Work out the finished part from the listing and answer in its coordinate system (mm). A direction names the side the tool comes from. Coordinates: 2 decimals unless noted, no trailing zeros. Order: outer loops, then holes, each group sorted by start corner. A loop starts at its lowest first (then second) coordinate and runs counter-clockwise, first axis right, second up. Notation, with made-up numbers: M 61.5,17.5 L 88.5,17.5 A10 ccw 88.5,36.5 Z; hole C 33.25,-7.75 d11. An arc over 180 degrees is marked long. Use a Markdown table: item, result.
from build123d import *

# Parameters (mm, degrees)
SKETCH1_R           = 3.8
SKETCH1_R_2         = 7.5
SKETCH1_R_3         = 6
SKETCH1_W           = 28
SKETCH1_H           = 21
BOSS_EXTRUDE1_DEPTH = 3


with BuildPart() as part:
    # Sketch1 → Boss-Extrude1 (new body)
    with BuildSketch(Plane.XY):
        with BuildLine():
            Line((-44.907534458, -41.831082964), (-44.907534458, -37.831082964))
            Line((-44.907534458, -37.831082964), (-74.907534458, -37.831082964))
            Line((-74.907534458, -37.831082964), (-77.907534458, -37.831082964))
            Line((-77.907534458, -37.831082964), (-77.907534458, 35.317270492))
            ThreePointArc((-77.907534458, 35.317270492), (-78.146852772, 36.26595379), (-78.807534458, 36.987599801))
            ThreePointArc((-78.807534458, 36.987599801), (-78.73201274, 48.728946501), (-68.036732481, 43.883752382))
            ThreePointArc((-68.036732481, 43.883752382), (-67.363200969, 42.667177293), (-66.059360488, 42.183752382))
            Line((-66.059360488, 42.183752382), (77.553779546, 42.183752382))
            Line((77.553779546, 42.183752382), (77.553779546, -37.831082964))
            Line((77.553779546, -37.831082964), (45.092465542, -37.831082964))
            Line((45.092465542, -37.831082964), (45.092465542, -41.831082964))
            Line((45.092465542, -41.831082964), (15.092465542, -41.831082964))
            Line((15.092465542, -41.831082964), (15.092465542, -37.831082964))
            Line((15.092465542, -37.831082964), (-14.907534458, -37.831082964))
            Line((-14.907534458, -37.831082964), (-14.907534458, -41.831082964))
            Line((-14.907534458, -41.831082964), (-44.907534458, -41.831082964))
        make_face()
        with Locations((-74.957534458, 42.833752382)):
            Circle(SKETCH1_R, mode=Mode.SUBTRACT)
        with Locations((-55.663947073, 16.489262872)):
            Circle(SKETCH1_R_2, mode=Mode.SUBTRACT)
        with Locations((-30.663947073, 16.489262872)):
            Circle(SKETCH1_R_2, mode=Mode.SUBTRACT)
        with Locations((-5.663947073, 16.489262872)):
            Circle(SKETCH1_R_2, mode=Mode.SUBTRACT)
        with Locations((54.950876551, -17.44070313)):
            Circle(SKETCH1_R_3, mode=Mode.SUBTRACT)
        with Locations((53.477773965, 15.276803872)):
            Rectangle(SKETCH1_W, SKETCH1_H, mode=Mode.SUBTRACT)
    extrude(amount=BOSS_EXTRUDE1_DEPTH)


solid = part.part
(1) Straight lines are drawn through the part: L1, parallel to Y at x = 40, z = 2.05; L2, parallel to X at y = 21, z = 1.7; L3, parallel to X at y = 20.5, z = 0.35. For each, find the intervals that lie inside material, in ascending order.
Conclusion:
| item | result |
|---|---|
| L1 | -41.83 to 4.78, 25.78 to 42.18 |
| L2 | -77.91 to -61.66, -49.67 to -36.66, -24.67 to -11.66, 0.33 to 39.48, 67.48 to 77.55 |
| L3 | -77.91 to -62, -49.33 to -37, -24.33 to -12, 0.67 to 39.48, 67.48 to 77.55 |
(2) Determine the mould class of faces 4 (the flat face through (53, 4.777, 1)), 5 (the cylindrical face through (-48.51, 18.74, 1.48)), 6 (the flat face through (-77.908, -2, 1)), 7 (the flat face through (62, -37.831, 1)) for opening direction Y: pulls with the +Y half, pulls with the -Y half, needs draft (parallel to the pull), parting line crosses it, or undercut.
Conclusion:
| item | result |
|---|---|
| face 4 | undercut |
| face 5 | undercut |
| face 6 | needs draft |
| face 7 | pulls with the -Y half |
(3) A cutting plane is placed at B-B (x = -30). Determine the outline of the cut face in (y, z).
Conclusion:
| item | result |
|---|---|
| outline | M -41.83,0 L 9.02,0 L 9.02,3 L -41.83,3 Z; M 23.96,0 L 42.18,0 L 42.18,3 L 23.96,3 Z |
(4) A cutting plane is placed at A-A (y = 10.5). Determine the outline of the cut face in (x, z), then the cut area to 3 significant figures.
Conclusion:
| item | result |
|---|---|
| outline | M -77.91,0 L -60.18,0 L -60.18,3 L -77.91,3 Z; M -51.15,0 L -35.18,0 L -35.18,3 L -51.15,3 Z; M -26.15,0 L -10.18,0 L -10.18,3 L -26.15,3 Z; M -1.15,0 L 39.48,0 L 39.48,3 L -1.15,3 Z; M 67.48,0 L 77.55,0 L 77.55,3 L 67.48,3 Z |
| area | 301 mm2 |
(5) A cutting plane is placed at D-D (y = -19). Determine the outline of the cut face in (x, z).
Conclusion:
| item | result |
|---|---|
| outline | M -77.91,0 L 49.16,0 L 49.16,3 L -77.91,3 Z; M 60.74,0 L 77.55,0 L 77.55,3 L 60.74,3 Z |
(6) Given P1, Ø1.5, axis at y = 2, z = 1, coming from the -X side; P2, Ø12, axis at x = 47, y = 16.5, coming from the -Z side; P3, Ø1.5, axis at x = -5, z = 1.5, coming from the -Y side; P4, Ø1.5, axis at y = -39.5, z = 1, coming from the +X side, each flat-ended and moving along its own axis, determine where each tip first touches the part or whether it passes through.
Conclusion:
| item | result |
|---|---|
| P1 | x = -77.91 |
| P2 | through |
| P3 | y = -37.83 |
| P4 | x = 45.09 |
(7) A cutting plane is placed at C-C (z = 0.9). Determine the outline of the cut face in (x, y), then the cut area to 3 significant figures.
Conclusion:
| item | result |
|---|---|
| outline | M -78.81,36.99 A2 cw -77.91,35.32 L -77.91,-37.83 L -44.91,-37.83 L -44.91,-41.83 L -14.91,-41.83 L -14.91,-37.83 L 15.09,-37.83 L 15.09,-41.83 L 45.09,-41.83 L 45.09,-37.83 L 77.55,-37.83 L 77.55,42.18 L -66.06,42.18 A2 cw -68.04,43.88 A7 ccw long Z; hole C -74.96,42.83 d7.6; hole C -55.66,16.49 d15; hole C -30.66,16.49 d15; hole C -5.66,16.49 d15; hole M 39.48,4.78 L 67.48,4.78 L 67.48,25.78 L 39.48,25.78 Z; hole C 54.95,-17.44 d12 |
| area | 11,500 mm2 |
(8) Which of the six approach directions +Z, -Z, +X, -X, +Y, -Y give full straight-line access (tool end or side, diameter ignored) to faces 1 (the flat face through (45.092, -40, 1)), 2 (the flat face through (67.478, 15, 1)), 3 (the flat face through (-14.908, -40, 1))?
Conclusion:
| item | result |
|---|---|
| face 1 | +Z, -Z, +X, -Y |
| face 2 | +Z, -Z |
| face 3 | +Z, -Z, -Y |
